```python
from build123d import *

# Parameters (mm, degrees)
SKETCH1_R               = 2.4
BOSS_EXTRUDE1_DEPTH     = 3
BOSS_EXTRUDE2_DEPTH     = 15.51
CUT_EXTRUDE1_DEPTH      = 5.31
CUT_EXTRUDE1_DEPTH_BACK = 5.31
SKETCH4_R               = 3.01
BOSS_EXTRUDE3_DEPTH     = 5.06
SKETCH5_R               = 0.925
SKETCH5_R_2             = 0.7
BOSS_EXTRUDE4_DEPTH     = 0.8
SKETCH6_R               = 0.823117729
BOSS_EXTRUDE5_DEPTH     = 5
CUT_EXTRUDE2_DEPTH      = 10


with BuildPart() as part:
    # Sketch1 → Boss-Extrude1 (new body)
    with BuildSketch(Plane.XY):
        Circle(SKETCH1_R)
    extrude(amount=BOSS_EXTRUDE1_DEPTH)

    # Sketch2 → Boss-Extrude2 (add)
    with BuildSketch(Plane.XY.offset(3)):
        with BuildLine():
            Line((4.31, 0), (4.31, -13.34))
            ThreePointArc((4.31, -13.34), (0, -17.65), (-4.31, -13.34))
            Line((-4.31, -13.34), (-4.31, 0))
            ThreePointArc((-4.31, 0), (0, 4.31), (4.31, 0))
        make_face()
    extrude(amount=BOSS_EXTRUDE2_DEPTH)

    # Sketch3 → Cut-Extrude1 (cut, two sides)
    with BuildSketch(Plane(origin=(0, 0, 0), x_dir=(0, 0, -1), z_dir=(1, 0, 0))) as cut_extrude1_sk:
        Polygon((-18.51, 4.31), (-15.55, 4.31), (-15.55, -5.79), (-18.51, -8.3), align=None)
    extrude(amount=CUT_EXTRUDE1_DEPTH, mode=Mode.SUBTRACT)
    extrude(cut_extrude1_sk.sketch, amount=-CUT_EXTRUDE1_DEPTH_BACK, mode=Mode.SUBTRACT)

    # Sketch4 → Boss-Extrude3 (add)
    with BuildSketch(Plane.XY.offset(18.51)):
        with Locations((0, -13.34)):
            Circle(SKETCH4_R)
    extrude(amount=BOSS_EXTRUDE3_DEPTH)

    # Sketch5 → Boss-Extrude4 (add)
    with BuildSketch(Plane(origin=(0, 0, 8.63), x_dir=(-1, 0, 0), z_dir=(0, 0, -1))):
        with BuildLine():
            Line((-3.31, 7.33), (3.31, 7.33))
            ThreePointArc((3.31, 7.33), (4.017106781, 7.037106781), (4.31, 6.33))
            Line((4.31, 6.33), (4.31, -19.67))
            ThreePointArc((4.31, -19.67), (4.017106781, -20.377106781), (3.31, -20.67))
            Line((3.31, -20.67), (-3.31, -20.67))
            ThreePointArc((-3.31, -20.67), (-4.017106781, -20.377106781), (-4.31, -19.67))
            Line((-4.31, -19.67), (-4.31, 6.33))
            ThreePointArc((-4.31, 6.33), (-4.017106781, 7.037106781), (-3.31, 7.33))
        make_face()
        with Locations((0, 6.13)):
            Circle(SKETCH5_R, mode=Mode.SUBTRACT)
        with Locations((3, 5.79076381)):
            Circle(SKETCH5_R_2, mode=Mode.SUBTRACT)
        with Locations((-3, 5.79076381)):
            Circle(SKETCH5_R_2, mode=Mode.SUBTRACT)
        with Locations((3, -19.13076381)):
            Circle(SKETCH5_R_2, mode=Mode.SUBTRACT)
        with Locations((0, -19.47)):
            Circle(SKETCH5_R, mode=Mode.SUBTRACT)
        with Locations((-3, -19.13076381)):
            Circle(SKETCH5_R_2, mode=Mode.SUBTRACT)
    extrude(amount=-BOSS_EXTRUDE4_DEPTH)

    # Sketch6 → Boss-Extrude5 (add)
    with BuildSketch(Plane(origin=(0, 4.302344091, 3.64827151), x_dir=(1, 0, 0), z_dir=(0, 0.7627017, 0.646750428))):
        with Locations((0, -17.550441075)):
            Circle(SKETCH6_R)
    extrude(amount=BOSS_EXTRUDE5_DEPTH)

    # Sketch7 → Cut-Extrude2 (cut)
    with BuildSketch(Plane(origin=(0, 0, 8.63), x_dir=(-1, 0, 0), z_dir=(0, 0, -1))):
        with BuildLine():
            Line((2.313724821, -18.992827668), (1.90235458, -21.039522477))
            Line((1.90235458, -21.039522477), (5.963625728, -21.039522477))
            Line((5.963625728, -21.039522477), (5.695977486, -18.025570536))
            Line((5.695977486, -18.025570536), (2.852857547, -18.446403453))
            ThreePointArc((2.852857547, -18.446403453), (2.491968028, -18.629511021), (2.313724821, -18.992827668))
        make_face()
    extrude(amount=-CUT_EXTRUDE2_DEPTH, mode=Mode.SUBTRACT)


solid = part.part
```
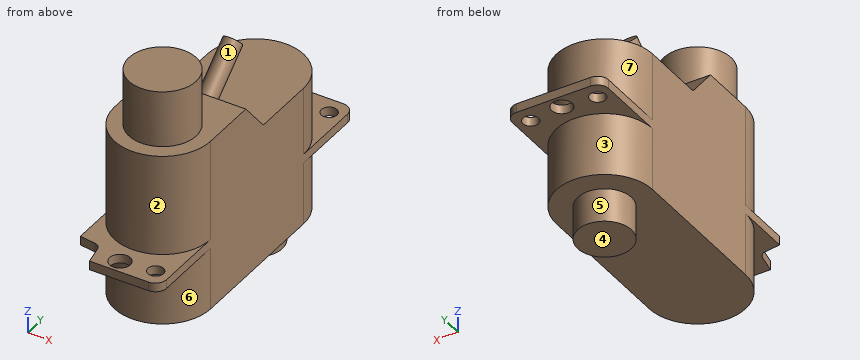
Check sheet for the modelled part. Datum: model origin and axes. Units: mm. Face numbers are marked on the shaded views. A direction names the side the tool comes from. Coordinates: 2 decimals unless noted, no trailing zeros. Order: outer loops, then holes, each group sorted by start corner. A loop starts at its lowest first (then second) coordinate and runs counter-clockwise, first axis right, second up. Notation, with made-up numbers: M 78,44 L 105,44 A24 ccw 105,69 Z; hole C 65,27 d1. An arc over 180 degrees is marked long. Write each question's results on one line, items separated by ' | '. Start each with the question number.
1. Cross-section at B-B on x = -1.5. Record the cut outline in (y, z).
2. Access from +Z, -Z, +X, -X, +Y, -Y to the whole of each face (thin tool, end or side, straight path). Record for the marked faces 5, 6 and 7.
3. Material ranges on probe 1 along Y at (x, z) = (3, 9.15); probe 2 along Y at (x, z) = (0, 9) (3 decimals); probe 3 along Z at (x, y) = (-1.25, -12), recorded low to high.
4. Mould release check, pull along Y, two halves, no side actions. Record for the marked faces 1, 2, 3 and 4: +Y half, -Y half, draft (parallel to the pull), parting line (faces both ways), or undercut.
5. Cross-section at C-C on z = 5. Record the cut outline in (x, y), and give its area (3 significant figures).
6. Cross-section at A-A on x = 0. State how many separate pieces and enclosed holes the cut face has, and give its area (3 significant figures).
7. Go/stop test with flat-tipped pins: P1, Ø2, axis at x = -2, y = 4, coming from the +Z side; P2, Ø1.6, axis at x = -3, y = 5.79, coming from the -Z side; P3, Ø4, axis at x = -2, z = 14.5, coming from the +Y side. Record where each tip stops, or that it passes through.
Checks:
1) outline: M -20.67,8.63 L -17.38,8.63 L -17.38,3 L -1.87,3 L -1.87,0 L 1.87,0 L 1.87,3 L 4.04,3 L 4.04,8.63 L 7.33,8.63 L 7.33,9.43 L 4.04,9.43 L 4.04,15.55 L -5.79,15.55 L -8.3,18.51 L -10.73,18.51 L -10.73,23.57 L -15.95,23.57 L -15.95,18.51 L -17.38,18.51 L -17.38,9.43 L -20.67,9.43 Z
2) face 5: -Z | face 6: -Z, -Y | face 7: +Z, +Y
3) probe 1: y = -20.67 to -19.83, -18.43 to 5.09, 6.49 to 7.33 | probe 2: y = -20.67 to -20.395, -18.545 to 5.205, 7.055 to 7.33 | probe 3: z = 3 to 23.57
4) face 1: undercut | face 2: -Y half | face 3: +Y half | face 4: draft
5) outline: M -4.31,-13.34 A4.31 ccw 4.31,-13.34 L 4.31,0 A4.31 ccw -4.31,0 Z | area: 173 mm²
6) separate pieces: 3 | enclosed holes: 0 | area: 362 mm²
7) P1: stops at z = 15.55 | P2: stops at z = 8.63 | P3: stops at y = 4.31
